Verification items for the finished model (mm, model axes). Face numbers are marked on the shaded views. Coordinates: 2 decimals unless noted, no trailing zeros. Loops run counter-clockwise (first coordinate to the right, second up) from the corner with the lowest first, then second, coordinate; pieces in that order, holes last. Notation, with made-up numbers: M 89,-16.75 L 108,-16.75 A32 cw 108,11.25 Z; hole C 15,21 d6. An arc over 180 degrees is marked long. Write item = value, one per line. Start each with the question number.
```python
from build123d import *

# Parameters (mm, degrees)
CONG_2_R = 0.5
CONG_3_R = 0.5


with BuildPart() as part:
    # Esquisse1 → Révolution1 (revolve)
    with BuildSketch(Plane.XY, mode=Mode.PRIVATE) as r_volution1_sk:
        Polygon((-9.5, -3), (-9.5, 3), (-7.5, 3), (-7.146446609, 2.646446609), (-6.792893219, 3), (-4.5, 3), (-4.5, -3), (-6.792893219, -3), (-7.146446609, -2.646446609), (-7.5, -3), align=None)
    revolve(r_volution1_sk.sketch.rotate(Axis((0, 0, 0), (0, 1, 0)), 270), axis=Axis((0, 0, 0), (0, 1, 0)))

    # Congé2
    cong_2_edges = [part.edges().sort_by_distance(p)[0] for p in [
        (0, 3, 6.792893219),
        (0, -3, 6.792893219),
    ]]
    fillet(cong_2_edges, radius=CONG_2_R)

    # Congé3
    cong_3_edges = [part.edges().sort_by_distance(p)[0] for p in [
        (0, 3, 9.5),
        (0, -3, 9.5),
    ]]
    fillet(cong_3_edges, radius=CONG_3_R)


solid = part.part
```
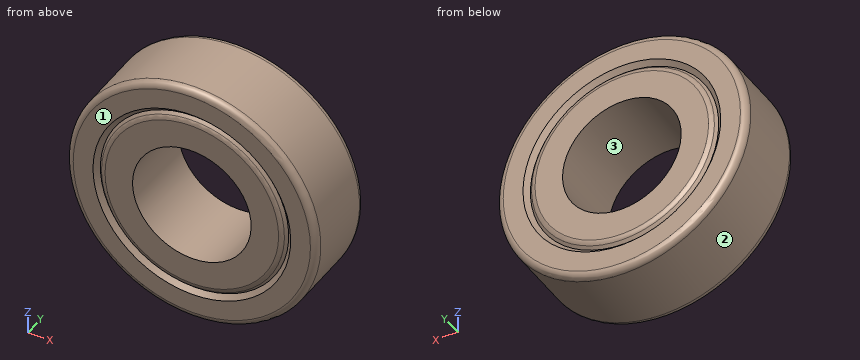
Q1. Gauge pin test, flat ends, axial feed: pin 1 (1.5 mm diameter, centred on y = 1.5, z = -1, fed in from -X); pin 2 (1.5 mm diameter, centred on y = 2, z = -2.5, fed in from +X); pin 3 (1 mm diameter, centred on x = -2.5, y = 2, fed in from +Z). Record the tip position at first contact, or that the pin passes through.
Q2. Sectioned sample at C-C on y = 1.25. Record the cut outline in (x, z), plus the area to 3 significant figures.
Q3. Scan lines: L1, parallel to X at y = 0.95, z = 0; L2, parallel to X at y = -1.05, z = -0.75; L3, parallel to Z at x = 1.5, y = 2.4. Record each from-to range of solid material in increasing order. Write a range as [from, to].
Q4. Sectioned sample at B-B on z = 0. Record the cut outline in (x, y).
Q5. Sectioned sample at A-A on x = 0. Record the cut outline in (y, z).
Q6. Mould release check, pull along Z, two halves, no side actions. Record for the marked faces 1, 2 and 3: +Z half, -Z half, draft (parallel to the pull), parting line (faces both ways), or undercut.
Solutions:
q1.pin_1 = -9.5
q1.pin_2 = 9.34
q1.pin_3 = 9.29
q2.outline = C 0,0 d19; hole C 0,0 d9
q2.area = 220 mm²
q3.L1 = [-9.5, -4.5], [4.5, 9.5]
q3.L2 = [-9.47, -4.44], [4.44, 9.47]
q3.L3 = [-9.38, -4.24], [4.24, 9.38]
q4.outline = M -9.5,-2.5 A0.5 ccw -9,-3 L -7.5,-3 L -7.15,-2.65 L -6.94,-2.85 A0.5 ccw -6.59,-3 L -4.5,-3 L -4.5,3 L -6.59,3 A0.5 ccw -6.94,2.85 L -7.15,2.65 L -7.5,3 L -9,3 A0.5 ccw -9.5,2.5 Z; M 4.5,-3 L 6.59,-3 A0.5 ccw 6.94,-2.85 L 7.15,-2.65 L 7.5,-3 L 9,-3 A0.5 ccw 9.5,-2.5 L 9.5,2.5 A0.5 ccw 9,3 L 7.5,3 L 7.15,2.65 L 6.94,2.85 A0.5 ccw 6.59,3 L 4.5,3 Z
q5.outline = M -3,-9 A0.5 ccw -2.5,-9.5 L 2.5,-9.5 A0.5 ccw 3,-9 L 3,-7.5 L 2.65,-7.15 L 2.85,-6.94 A0.5 ccw 3,-6.59 L 3,-4.5 L -3,-4.5 L -3,-6.59 A0.5 ccw -2.85,-6.94 L -2.65,-7.15 L -3,-7.5 Z; M -3,4.5 L 3,4.5 L 3,6.59 A0.5 ccw 2.85,6.94 L 2.65,7.15 L 3,7.5 L 3,9 A0.5 ccw 2.5,9.5 L -2.5,9.5 A0.5 ccw -3,9 L -3,7.5 L -2.65,7.15 L -2.85,6.94 A0.5 ccw -3,6.59 Z
q6.face_1 = draft
q6.face_2 = parting line
q6.face_3 = undercut
